Design review of the part built by this model. Coordinates are the model's own, in mm. Face numbers are marked on the shaded views. A direction names the side the tool comes from. Coordinates: 2 decimals unless noted, no trailing zeros. Order: outer loops, then holes, each group sorted by start corner. A loop starts at its lowest first (then second) coordinate and runs counter-clockwise, first axis right, second up. Notation, with made-up numbers: M 85,-16 L 91,-16 A10 cw 91,3 Z; hole C 54.5,-18.75 d2. An arc over 180 degrees is marked long. Answer as a JSON object with one key per item and string values.
from build123d import *

# Parameters (mm, degrees)
F0_R     = 4
F1_DEPTH = 15
F3_DEPTH = 10


with BuildPart() as f1:
    # F0 (on Top) → F1 (new body)
    with BuildSketch(Plane.XY):
        Circle(F0_R)
    extrude(amount=F1_DEPTH)

    # F2 (on face) → F3 (join)
    with BuildSketch(Plane.XY.offset(15)):
        with BuildLine():
            Line((0, -7.05), (0, 0))
            Line((0, 0), (0, 7.05))
            Line((0, 7.05), (-1.975, 7.05))
            ThreePointArc((-1.975, 7.05), (-9.025, 0), (-1.975, -7.05))
            Line((-1.975, -7.05), (0, -7.05))
        make_face()
        with BuildLine():
            Line((0, 7.05), (0, 0))
            Line((0, 0), (0, -7.05))
            Line((0, -7.05), (1.975, -7.05))
            ThreePointArc((1.975, -7.05), (9.025, 0), (1.975, 7.05))
            Line((1.975, 7.05), (0, 7.05))
        make_face()
    extrude(amount=F3_DEPTH)


solid = f1.part
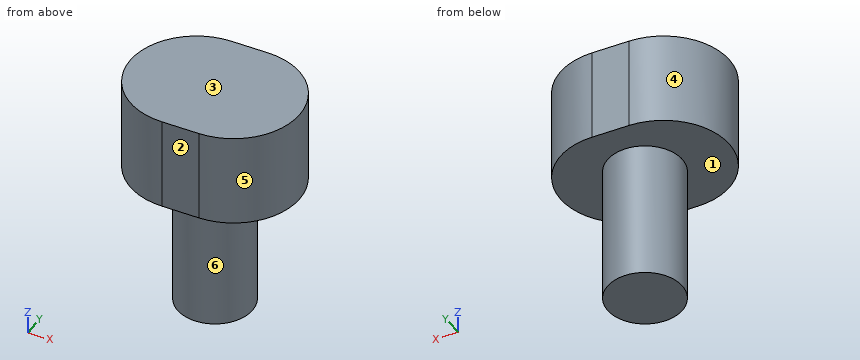
1) Mouldability with a two-part tool opening along X and no side actions: class the marked faces 3, 4, 5 and 6 as released by +X, released by -X, zero draft, split by the parting line, or undercut.
Taken from the geometry:
{"face 3": "zero draft", "face 4": "released by -X", "face 5": "released by +X", "face 6": "split by the parting line"}
2) Insertion check: pin 1 Ø2 at (x, z) = (1, 8) entering from +Y; pin 2 Ø3 at (y, z) = (-0.5, 12.5) entering from +X; pin 3 Ø1.5 at (x, z) = (-1.5, 3.5) entering from +Y. Each pin has a flat end and moves straight along its axis. Give the tip position at first contact, or say it passes through.
Taken from the geometry:
{"pin 1": "stops at y = 4", "pin 2": "stops at x = 4", "pin 3": "stops at y = 3.93"}
3) Tool access review of the marked faces 1 and 2: name each direction out of +Z, -Z, +X, -X, +Y, -Y from which nothing blocks a thin tool from reaching the whole face with its end or side.
Taken from the geometry:
{"face 1": "-Z", "face 2": "+Z, -Z, +X, -X, -Y"}
4) Add section B-B (x = 0). State the section outline as (y, z) points, and give its area (3 significant figures).
Taken from the geometry:
{"outline": "M -7.05,15 L -4,15 L -4,0 L 4,0 L 4,15 L 7.05,15 L 7.05,25 L -7.05,25 Z", "area": "261 mm2"}
5) Add section D-D (z = 20). State the section outline as (x, y) points (3 decimals).
Taken from the geometry:
{"outline": "M -1.975,-7.05 L 1.975,-7.05 A7.05 ccw 1.975,7.05 L -1.975,7.05 A7.05 ccw Z"}
6) Add section C-C (z = 7.5). State the section outline as (x, y) points.
Taken from the geometry:
{"outline": "C 0,0 d8"}
7) To check wall thickness, follow L1, parallel to Z at x = 7.25, y = 3.5; L2, parallel to X at y = 2.25, z = 3.5; L3, parallel to Y at x = 3.5, z = 6. State the ranges of each line that lie inside material, in increasing order.
Taken from the geometry:
{"L1": "z = 15 to 25", "L2": "x = -3.31 to 3.31", "L3": "y = -1.94 to 1.94"}
8) Add section A-A (y = 0). State the section outline as (x, z) points (3 decimals), and give its area (4 significant figures).
Taken from the geometry:
{"outline": "M -9.025,15 L -4,15 L -4,0 L 4,0 L 4,15 L 9.025,15 L 9.025,25 L -9.025,25 Z", "area": "300.5 mm2"}
